from build123d import *

# Parameters (mm, degrees)
F0_W     = 400
F0_H     = 150
F1_DEPTH = 12.5
F2_SIZE  = 24.99999


# Not quite as in the source:
# - a fillet or chamfer is up to 0.001 mm smaller than in the source, because OpenCascade refuses the exact size


with BuildPart() as f1:
    # F0 (on Top) → F1 (new body, symmetric)
    with BuildSketch(Plane.XY):
        Rectangle(F0_W, F0_H)
    extrude(amount=F1_DEPTH, both=True)

    # F2 (size 25 in the source; OpenCascade refuses exactly that, so slightly less here)
    f2_edges = [f1.edges().sort_by_distance(p)[0] for p in [
        (0, 75, -12.5),
        (-200, 0, -12.5),
        (0, -75, -12.5),
    ]]
    chamfer(f2_edges, length=F2_SIZE)


solid = f1.part
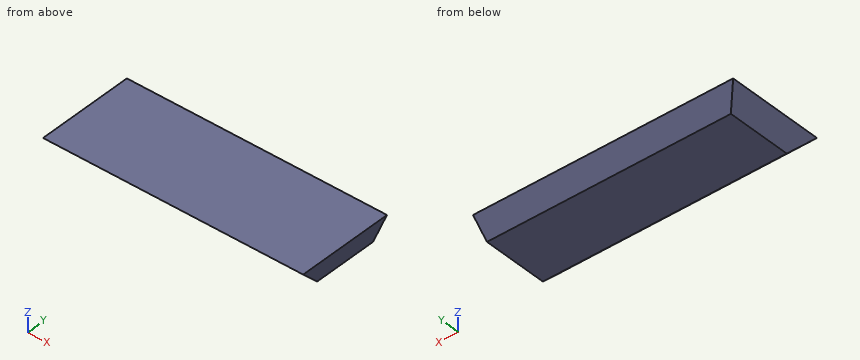
CAD build for the part. Positions are in the model's coordinates, mm. Round coordinates to 2 decimals unless told otherwise and drop trailing zeros. Loops run counter-clockwise (first coordinate to the right, second up) from the corner with the lowest first, then second, coordinate; pieces in that order, holes last.
(1) Wall check: line 1 along Y through (x, z) = (156, 5); line 2 along Y through (x, z) = (18.5, -1); line 3 along Z through (x, y) = (-27, 60). Give the ranges that are in metal, low to high.
(2) Cut at C-C (z = -8.75). Give the cut face in (x, y), plus the area to 3 significant figures.
(3) Drop flat-ended pins along their axis: pin 1 (1.5 mm diameter, centred on x = -128.5, z = -9, fed in from +Y); pin 2 (6 mm diameter, centred on y = -2, z = -0.5, fed in from -X); pin 3 (1.5 mm diameter, centred on y = 59.5, z = -4.5, fed in from +X); pin 4 (6 mm diameter, centred on x = 40.5, z = 3.5, fed in from +Y). Give the stop position or say it passes through.
Findings below:
1. line 1: y = -67.5 to 67.5
1. line 2: y = -61.5 to 61.5
1. line 3: z = -2.5 to 12.5
2. outline: (-178.75, -53.75) - (200, -53.75) - (200, 53.75) - (-178.75, 53.75) - close
2. area: 40,700 mm2
3. pin 1: stops at y = 54.25
3. pin 2: stops at x = -190
3. pin 3: passes through
3. pin 4: stops at y = 69
